Here's how the part is built. I have some questions about the finished solid (model axes, mm). A direction names the side the tool comes from. Give positions to 0.01 mm unless a question says otherwise; leave off trailing zeros. Write each loop counter-clockwise with the first axis right and the second up, starting at its lowest first coordinate (ties: lowest second). Pieces come first, ordered by that corner, then holes. Notation, with made-up numbers: (58, 62) - (66, 62) arc R20 cw to (66, 66) - close; hole circle Ø11 at (25.25, -38). An arc over 180 degrees is marked (long way). One line per item, written item: value. Start each with the question number.
1) I'm going to push flat-ended pins straight in: P1, Ø4, axis at y = 12.5, z = 26, coming from the -X side; P2, Ø5, axis at x = 17, z = 31, coming from the +Y side (3 decimals); P3, Ø6, axis at y = 5, z = 20, coming from the +X side. Where does each tip first touch, or does it pass through?
2) Imagine slicing it at D-D on x = 0. Count the separate pieces of the cut face and the enclosed holes in it, plus the area to 3 significant figures.
3) Imagine slicing it at A-A on y = 12. Write out the boundary of the cut face in (x, z), plus the area to 3 significant figures.
4) On a 3-axis mill with a long thin cutter (end or side, diameter ignored), from which of +Z, -Z, +X, -X, +Y, -Y can I reach the whole of each face in a straight line? I mean faces 1 (the flat face through (9.929, 13, 25)), 2 (the flat face through (0, 10, 22.772)), 3 (the flat face through (0, 15.575, -24)), 4 (the flat face through (-10.229, 13, -25)). Say none if no direction works.
5) Please list where these lines run through material, in increasing order: L1, parallel to Y at x = 9.5, z = 24.5 (3 decimals); L2, parallel to Y at x = 14, z = -32.5 (3 decimals); L3, parallel to Z at x = 3.5, y = 9. Write a range as [from, to].
6) We'd pull the mould along X, two halves only. Please class faces 5 (the flat face through (-31, 3, 1)), 6 (the cylindrical face through (0.07, 0.71, -39.5)), 7 (the flat face through (0, 15.575, 24)), 8 (the cylindrical face through (10.531, 5.145, 25.445)): +X half, -X half, draft (parallel to the pull), parting line (faces both ways), or undercut.
from build123d import *

# Parameters (mm, degrees)
SKETCH1_W           = 62
SKETCH1_H           = 76
BOSS_EXTRUDE1_DEPTH = 4.575
SKETCH11_W          = 66
SKETCH11_H          = 80
BOSS_EXTRUDE5_DEPTH = 1.4
BOSS_EXTRUDE3_DEPTH = 1.4
CUT_EXTRUDE3_REACH  = 57.092
SKETCH12_R          = 1.5
FILLET1_R           = 1.4
SKETCH21_W          = 20.158508521
SKETCH21_H          = 5
BOSS_EXTRUDE8_DEPTH = 15
SKETCH33_W          = 3
SKETCH33_H          = 2
CUT_EXTRUDE7_DEPTH  = 25
FILLET2_R           = 2


with BuildPart() as part:
    # Sketch1 → Boss-Extrude1 (new body)
    with BuildSketch(Plane(origin=(0, 0, 0), x_dir=(1, 0, 0), z_dir=(0, 1, 0))):
        Rectangle(SKETCH1_W, SKETCH1_H)
    extrude(amount=BOSS_EXTRUDE1_DEPTH)

    # Sketch11 → Boss-Extrude5 (add)
    with BuildSketch(Plane(origin=(0, 0, 0), x_dir=(-1, 0, 0), z_dir=(0, -1, 0))):
        Rectangle(SKETCH11_W, SKETCH11_H)
    extrude(amount=-BOSS_EXTRUDE5_DEPTH)

    # Sketch4 → Boss-Extrude3 (add)
    with BuildSketch(Plane(origin=(0, 0, 0), x_dir=(1, 0, 0), z_dir=(0, 1, 0))):
        with BuildLine():
            Line((-8, -40), (8, -40))
            ThreePointArc((8, -40), (6.211145618, -40.422291236), (4.8, -41.6))
            ThreePointArc((4.8, -41.6), (0, -44), (-4.8, -41.6))
            ThreePointArc((-4.8, -41.6), (-6.211145618, -40.422291236), (-8, -40))
        make_face()
    boss_extrude3 = extrude(amount=BOSS_EXTRUDE3_DEPTH)

    # Sketch12 → Cut-Extrude3 (cut, up to next)
    with BuildSketch(Plane(origin=(0, 1.4, 0), x_dir=(1, 0, 0), z_dir=(0, 1, 0)), mode=Mode.PRIVATE) as cut_extrude3_sk1:
        with Locations(Location((0, -41, 0), (0, 0, 270))):
            Circle(SKETCH12_R)
    cut_extrude3_tool1 = extrude(cut_extrude3_sk1.sketch, amount=-CUT_EXTRUDE3_REACH, mode=Mode.PRIVATE) & part.part
    cut_extrude3 = cut_extrude3_tool1.solids().sort_by_distance((0, 1.4, 41))[0]
    add(cut_extrude3, mode=Mode.SUBTRACT)

    # Mirror1: Boss-Extrude3, Cut-Extrude3 across plane
    add(boss_extrude3.mirror(Plane.XY))
    add(cut_extrude3.mirror(Plane.XY), mode=Mode.SUBTRACT)

    # Fillet1
    fillet1_edges = [part.edges().sort_by_distance(p)[0] for p in [
        (20.5, 0, -40),
        (6.211145618, 0, -40.422291236),
        (0, 0, -44),
        (-6.211145618, 0, -40.422291236),
        (-20.5, 0, -40),
        (-33, 0, 0),
        (-20.5, 0, 40),
        (-6.211145618, 0, 40.422291236),
        (0, 0, 44),
        (6.211145618, 0, 40.422291236),
        (20.5, 0, 40),
        (33, 0, 0),
    ]]
    fillet(fillet1_edges, radius=FILLET1_R - 0.0001)  # a hair under: the kernel refuses the full size

    # Sketch21 → Boss-Extrude8 (add)
    with BuildSketch(Plane(origin=(0, 4.575, 0), x_dir=(1, 0, 0), z_dir=(0, 1, 0))):
        with Locations((-0.149821344, -25.272162816)):
            Rectangle(SKETCH21_W, SKETCH21_H)
    boss_extrude8 = extrude(amount=BOSS_EXTRUDE8_DEPTH)

    # Sketch33 → Cut-Extrude7 (cut)
    with BuildSketch(Plane(origin=(9.929432917, 0, 0), x_dir=(0, 0, -1), z_dir=(1, 0, 0))):
        with Locations((-24.272162816, 16.575)):
            Rectangle(SKETCH33_W, SKETCH33_H)
    cut_extrude7 = extrude(amount=-CUT_EXTRUDE7_DEPTH, mode=Mode.SUBTRACT)

    # Mirror2: Boss-Extrude8, Cut-Extrude7 across plane
    add(boss_extrude8.mirror(Plane.XY))
    add(cut_extrude7.mirror(Plane.XY), mode=Mode.SUBTRACT)

    # Fillet2
    fillet2_edges = [part.edges().sort_by_distance(p)[0] for p in [
        (-10.229075604, 4.575, 25.272162816),
        (-0.149821344, 4.575, 27.772162816),
        (9.929432917, 4.575, 25.272162816),
        (9.929432917, 4.575, -25.272162816),
        (-10.229075604, 4.575, -25.272162816),
        (-0.149821344, 4.575, -27.772162816),
    ]]
    fillet(fillet2_edges, radius=FILLET2_R)


solid = part.part
Numbers:
1. P1: x = -10.23
1. P2: y = 4.575
1. P3: x = 31
2. separate pieces: 3
2. enclosed holes: 0
2. area: 495 mm^2
3. outline: (-10.23, -27.77) - (9.93, -27.77) - (9.93, -22.77) - (-10.23, -22.77) - close; (-10.23, 22.77) - (9.93, 22.77) - (9.93, 27.77) - (-10.23, 27.77) - close
3. area: 202 mm^2
4. face 1: +Z, -Z, +X, +Y
4. face 2: +X, -X, +Y
4. face 3: +X, -X
4. face 4: +Z, -Z, -X, +Y
5. L1: [0, 15.575], [17.575, 19.575]
5. L2: [0, 4.575]
5. L3: [-27.77, -22.77], [22.77, 27.77]
6. face 5: -X half
6. face 6: undercut
6. face 7: draft
6. face 8: +X half
